Verification items for the finished model (mm, model axes). A direction names the side the tool comes from. Give positions to 0.01 mm unless a question says otherwise; leave off trailing zeros. Write each loop counter-clockwise with the first axis right and the second up, starting at its lowest first coordinate (ties: lowest second). Pieces come first, ordered by that corner, then holes. Notation, with made-up numbers: (-8.75, -28.5) -> (5.25, -28.5) arc R14 cw to (5.25, -23.5) -> close; hole circle Ø7 at (-23.5, -25.75). An arc over 180 degrees is marked (long way). Use CSV: the item, a comma, the result in double quotes. Start each with the question number.
```python
from build123d import *

# Parameters (mm, degrees)
SKETCH1_W           = 250
SKETCH1_H           = 180
BOSS_EXTRUDE1_DEPTH = 10
CUT_EXTRUDE1_DEPTH  = 10
CIRPATTERN1_COUNT   = 4


with BuildPart() as part:
    # Sketch1 → Boss-Extrude1 (new body)
    with BuildSketch(Plane.XY):
        with Locations((75, -50)):
            Rectangle(SKETCH1_W, SKETCH1_H)
    extrude(amount=BOSS_EXTRUDE1_DEPTH)

    # Sketch2 → Cut-Extrude1 (cut)
    with BuildSketch(Plane.XY.offset(10)):
        with BuildLine():
            Line((70.5, -22.5), (70.5, -57.5))
            ThreePointArc((70.5, -57.5), (65, -63), (59.5, -57.5))
            Line((59.5, -57.5), (59.5, -22.5))
            ThreePointArc((59.5, -22.5), (65, -17), (70.5, -22.5))
        make_face()
    cut_extrude1 = extrude(amount=-CUT_EXTRUDE1_DEPTH, mode=Mode.SUBTRACT)

    # CirPattern1: Cut-Extrude1 ×4 about axis
    cirpattern1_axis = Axis((105, -50, 0), (0, 0, 1))
    for i in range(1, CIRPATTERN1_COUNT):
        add(cut_extrude1.rotate(cirpattern1_axis, i * 360 / CIRPATTERN1_COUNT), mode=Mode.SUBTRACT)


solid = part.part
```
(1) Thickness scan on line 1 (X direction, y = -52, z = 8); line 2 (X direction, y = -25.5, z = 1.75); line 3 (Y direction, x = 122, z = 4.75). Record the ranges inside material, lowest first. Write a range as from..to.
(2) Set-up check for faces 1 (the face through (200, -51, 5)), 2 (the face through (145, -83, 5)): record each of +Z, -Z, +X, -X, +Y, -Y from which the full face is reachable in a straight line by a thin tool's end or side.
(3) Draft check along Y on faces 3 (the face through (115, -4.5, 5)), 4 (the face through (118, -90, 5)), 5 (the face through (73, -49, 10)), 6 (the face through (73, 40, 5)). Enter one of: released by +Y, released by -Y, zero draft, split by the parting line, or undercut.
(4) Section check A-A on x = 145. Record the cut outline in (y, z).
(5) Section check B-B on y = -74. Record the cut outline in (x, z).
(6) Section check C-C on z = 1.75. Record the cut outline in (x, y), then the cut area to 3 significant figures.
Data:
1,line 1,"x = -50..59.5, 70.5..139.5, 150.5..200"
1,line 2,"x = -50..59.5, 70.5..200"
1,line 3,"y = -140..-15.5, -4.5..40"
2,face 1,"+Z, -Z, +X, +Y, -Y"
2,face 2,"+Z, -Z"
3,face 3,"undercut"
3,face 4,"undercut"
3,face 5,"zero draft"
3,face 6,"released by +Y"
4,outline,"(-140, 0) -> (-83, 0) -> (-83, 10) -> (-140, 10) -> close; (-37, 0) -> (40, 0) -> (40, 10) -> (-37, 10) -> close"
5,outline,"(-50, 0) -> (139.5, 0) -> (139.5, 10) -> (-50, 10) -> close; (150.5, 0) -> (200, 0) -> (200, 10) -> (150.5, 10) -> close"
6,outline,"(-50, -140) -> (200, -140) -> (200, 40) -> (-50, 40) -> close; hole (59.5, -57.5) arc R5.5 ccw to (70.5, -57.5) -> (70.5, -22.5) arc R5.5 ccw to (59.5, -22.5) -> close; hole (77.5, -95.5) -> (112.5, -95.5) arc R5.5 ccw to (112.5, -84.5) -> (77.5, -84.5) arc R5.5 ccw to start; hole (97.5, -15.5) -> (132.5, -15.5) arc R5.5 ccw to (132.5, -4.5) -> (97.5, -4.5) arc R5.5 ccw to start; hole (139.5, -77.5) arc R5.5 ccw to (150.5, -77.5) -> (150.5, -42.5) arc R5.5 ccw to (139.5, -42.5) -> close"
6,area,"43,100 mm2"
